The listing builds one solid part. Answer for the finished solid, in the listing's coordinates (mm). Face numbers are marked on the shaded views. A direction names the side the tool comes from. Coordinates: 2 decimals unless noted, no trailing zeros. Loops run counter-clockwise (first coordinate to the right, second up) from the corner with the lowest first, then second, coordinate; pieces in that order, holes last. Notation, with made-up numbers: (52.25, 11.5) - (95.25, 11.5) arc R24 ccw to (95.25, 24.5) - close; hole circle Ø10 at (27.25, 25). An arc over 180 degrees is marked (long way). Use one line per item in the form item = value. Start each with the question number.
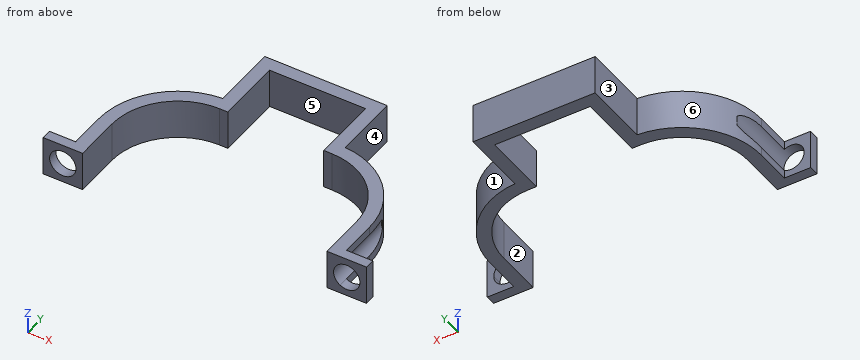
```python
from build123d import *

# Parameters (mm, degrees)
EXTRUDE_1_DEPTH          = 6
CUT_EXTRUDE_1_DEPTH      = 10
CUT_EXTRUDE_1_DEPTH_BACK = 10
SKETCH_2_R               = 2


with BuildPart() as part:
    # 스케치1 → 보스-돌출1 (new body)
    with BuildSketch(Plane.XY):
        with BuildLine():
            Line((31.75, 18.5), (33, 18.5))
            ThreePointArc((33, 18.5), (40.071067812, 15.571067812), (43, 8.5))
            Line((43, 8.5), (43, 1.5))
            Line((43, 1.5), (49, 1.5))
            Line((49, 1.5), (49, 3))
            Line((49, 3), (45, 3))
            Line((45, 3), (45, 8.5))
            ThreePointArc((45, 8.5), (41.746427842, 16.715838363), (33.75, 20.476539567))
            Line((33.75, 20.476539567), (33.75, 30.5))
            Line((33.75, 30.5), (15.25, 30.5))
            Line((15.25, 30.5), (15.25, 20.476539567))
            ThreePointArc((15.25, 20.476539567), (7.253572158, 16.715838363), (4, 8.5))
            Line((4, 8.5), (4, 3))
            Line((4, 3), (0, 3))
            Line((0, 3), (0, 1.5))
            Line((0, 1.5), (6, 1.5))
            Line((6, 1.5), (6, 8.5))
            ThreePointArc((6, 8.5), (8.928932188, 15.571067812), (16, 18.5))
            Line((16, 18.5), (17.25, 18.5))
            Line((17.25, 18.5), (17.25, 28.5))
            Line((17.25, 28.5), (31.75, 28.5))
            Line((31.75, 28.5), (31.75, 18.5))
        make_face()
    extrude(amount=EXTRUDE_1_DEPTH)

    # 스케치2 → 컷-돌출1 (cut, two sides: drawn at the far end of the back side and taken through both)
    with BuildSketch(Plane(origin=(0, 3, 0), x_dir=(1, 0, 0), z_dir=(0, 1, 0)).offset(-CUT_EXTRUDE_1_DEPTH_BACK)):
        with BuildLine():
            ThreePointArc((45, -4.732050808), (47, -4.732050808), (48, -3))
            ThreePointArc((48, -3), (47, -1.267949192), (45, -1.267949192))
            Line((45, -1.267949192), (45, -4.732050808))
        make_face()
        with BuildLine():
            Line((45, -4.732050808), (45, -1.267949192))
            ThreePointArc((45, -1.267949192), (44, -3), (45, -4.732050808))
        make_face()
        with Locations(Location((3, -3, 0), (0, 0, 60))):
            Circle(SKETCH_2_R)
    extrude(amount=CUT_EXTRUDE_1_DEPTH + CUT_EXTRUDE_1_DEPTH_BACK, mode=Mode.SUBTRACT)


solid = part.part
```
(1) A cutting plane is placed at D-D (y = 6.5). Determine the outline of the cut face in (x, z), then the cut area to 3 significant figures.
(2) A cutting plane is placed at B-B (x = 3). Determine the outline of the cut face in (y, z), then the cut area to 3 significant figures.
(3) Find the intervals of material crossed by probe 1 along X at (y, z) = (23.5, 5.5); probe 2 along X at (y, z) = (4.5, 5.25); probe 3 along Y at (x, z) = (16.5, 4.25), in increasing order. Write a range as from..to.
(4) A cutting plane is placed at A-A (y = 23.25). Determine the outline of the cut face in (x, z), then the cut area to 3 significant figures.
(5) Each of these flat-tipped pins is pushed along its axis until it touches: pin 1 Ø3 at (y, z) = (5.5, 3.5) entering from -X; pin 2 Ø2 at (x, z) = (48, 3.5) entering from +Y; pin 3 Ø3 at (x, z) = (24, 4) entering from -Y. Where does it stop, or does it pass through?
(6) Determine the mould class of the marked faces 1, 2 and 3 for opening direction X: +X half, -X half, draft (parallel to the pull), parting line (faces both ways), or undercut.
(7) A cutting plane is placed at C-C (z = 0.5). Determine the outline of the cut face in (x, y), then the cut area to 3 significant figures.
(8) For the marked faces 4, 5 and 6, determine the directions among +Z, -Z, +X, -X, +Y, -Y from which every point of the face is accessible in a straight line to the end or side of a thin tool.
Evaluation:
q1.outline = (4, 0) - (6, 0) - (6, 6) - (4, 6) - (4, 4.73) arc R2 cw to (4, 1.27) - close; (43, 0) - (45, 0) - (45, 1.27) arc R2 cw to (45, 4.73) - (45, 6) - (43, 6) - close
q1.area = 19.1 mm^2
q2.outline = (1.5, 0) - (3, 0) - (3, 1) - (1.5, 1) - close; (1.5, 5) - (3, 5) - (3, 6) - (1.5, 6) - close
q2.area = 3.00 mm^2
q3.probe_1 = 15.25..17.25, 31.75..33.75
q3.probe_2 = 4..6, 43..45
q3.probe_3 = 18.5..30.5
q4.outline = (15.25, 0) - (17.25, 0) - (17.25, 6) - (15.25, 6) - close; (31.75, 0) - (33.75, 0) - (33.75, 6) - (31.75, 6) - close
q4.area = 24.0 mm^2
q5.pin_1 = 4
q5.pin_2 = 3
q5.pin_3 = 28.5
q6.face_1 = +X half
q6.face_2 = undercut
q6.face_3 = -X half
q7.outline = (0, 1.5) - (6, 1.5) - (6, 8.5) arc R10 cw to (16, 18.5) - (17.25, 18.5) - (17.25, 28.5) - (31.75, 28.5) - (31.75, 18.5) - (33, 18.5) arc R10 cw to (43, 8.5) - (43, 1.5) - (49, 1.5) - (49, 3) - (45, 3) - (45, 8.5) arc R12 ccw to (33.75, 20.48) - (33.75, 30.5) - (15.25, 30.5) - (15.25, 20.48) arc R12 ccw to (4, 8.5) - (4, 3) - (0, 3) - close
q7.area = 183 mm^2
q8.face_4 = +Z, -Z, +X, +Y
q8.face_5 = +Z, -Z, -Y
q8.face_6 = +Z, -Z, -X, +Y
